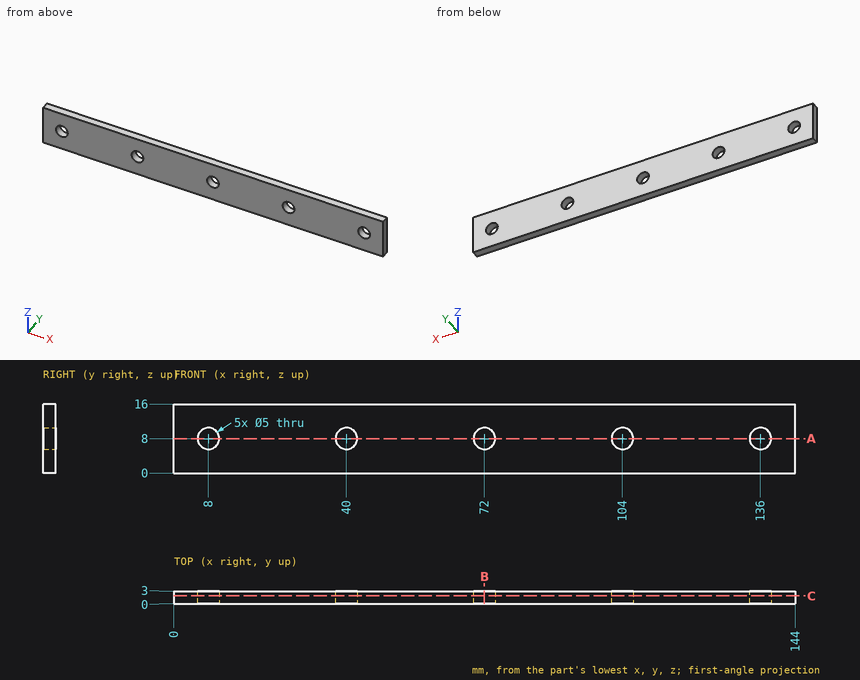
Check sheet for the drawn part. Datum: minimum x, y, z corner. Units: mm. Round coordinates to 2 decimals unless told otherwise and drop trailing zeros. Write each loop counter-clockwise with the first axis right and the second up, starting at its lowest first coordinate (ties: lowest second). Pieces come first, ordered by that corner, then holes. Notation, with made-up numbers: (72.25, 0) -> (105.25, 0) arc R18 ccw to (105.25, 32) -> close; hole circle Ø4 at (32.5, -7.5). An arc over 180 degrees is marked (long way). One line per item, written item: value. Start each with the question number.
(1) Scan lines: line 1 (Z direction, x = 8, y = 2.55); line 2 (X direction, y = 0.35, z = 6.25); line 3 (X direction, y = 1.35, z = 10.25). Record each from-to range of solid material in increasing order. Write a range as [from, to].
(2) Go/stop test with a flat-tipped pin: pin 1 Ø2 at (x, z) = (89.5, 5.5) entering from -Y. Record where the tip stops, or that it passes through.
(3) Cross-section at B-B, the plane x = 72. Record the cut outline in (y, z).
(4) Cross-section at C-C, the plane y = 1.85. Record the cut outline in (x, z), and give its area (3 significant figures).
(5) Cross-section at A-A, the plane z = 8. Record the cut outline in (x, y), and give its area (3 significant figures).
Answer:
1. line 1: [0, 5.5], [10.5, 16]
1. line 2: [0, 6.21], [9.79, 38.21], [41.79, 70.21], [73.79, 102.21], [105.79, 134.21], [137.79, 144]
1. line 3: [0, 6.91], [9.09, 38.91], [41.09, 70.91], [73.09, 102.91], [105.09, 134.91], [137.09, 144]
2. pin 1: y = 0
3. outline: (0, 0) -> (3, 0) -> (3, 5.5) -> (0, 5.5) -> close; (0, 10.5) -> (3, 10.5) -> (3, 16) -> (0, 16) -> close
4. outline: (0, 0) -> (144, 0) -> (144, 16) -> (0, 16) -> close; hole circle Ø5 at (8, 8); hole circle Ø5 at (40, 8); hole circle Ø5 at (72, 8); hole circle Ø5 at (104, 8); hole circle Ø5 at (136, 8)
4. area: 2,210 mm²
5. outline: (0, 0) -> (5.5, 0) -> (5.5, 3) -> (0, 3) -> close; (10.5, 0) -> (37.5, 0) -> (37.5, 3) -> (10.5, 3) -> close; (42.5, 0) -> (69.5, 0) -> (69.5, 3) -> (42.5, 3) -> close; (74.5, 0) -> (101.5, 0) -> (101.5, 3) -> (74.5, 3) -> close; (106.5, 0) -> (133.5, 0) -> (133.5, 3) -> (106.5, 3) -> close; (138.5, 0) -> (144, 0) -> (144, 3) -> (138.5, 3) -> close
5. area: 357 mm²
